The listing builds one solid part. Answer for the finished solid, in the listing's coordinates (mm). Face numbers are marked on the shaded views. A direction names the side the tool comes from. Coordinates: 2 decimals unless noted, no trailing zeros. Order: outer loops, then holes, each group sorted by start corner. A loop starts at its lowest first (then second) coordinate and runs counter-clockwise, first axis right, second up. Notation, with made-up numbers: (24.25, 67) -> (50.25, 67) arc R31 ccw to (50.25, 91) -> close; hole circle Ø1 at (60.25, 74). An arc over 180 degrees is marked (long way). Write each question's results on one line, items separated by ' | '. Start each with the question number.
(1) Given pin 1 (3 mm diameter, centred on y = -1, z = 15, fed in from +X); pin 2 (0.5 mm diameter, centred on x = -17, y = 13.5, fed in from +Z); pin 3 (1 mm diameter, centred on y = 14.5, z = 5.5, fed in from +X); pin 4 (2 mm diameter, centred on x = 19.5, y = -17.5, fed in from -Z), each flat-ended and moving along its own axis, determine where each tip first touches the part or whether it passes through.
(2) The part is cut by section B-B, the plane z = 1. Give the vertices of the cut face in (x, y).
(3) A tool of negligible diameter and unlimited length cuts with its end or side. For the marked faces 1 and 2, from which of +Z, -Z, +X, -X, +Y, -Y can it reach the whole face along a straight path? Write none if from no direction.
(4) The part is cut by section A-A, the plane z = 10.25. Count the separate pieces of the cut face and the enclosed holes in it, then the cut area to 3 significant figures.
(5) Straight lines are drawn through the part: L1, parallel to Y at x = 12, z = 13; L2, parallel to X at y = 19.5, z = 7.75; L3, parallel to Y at x = -3.5, z = 14.25. For each, find the intervals that lie inside material, in ascending order.
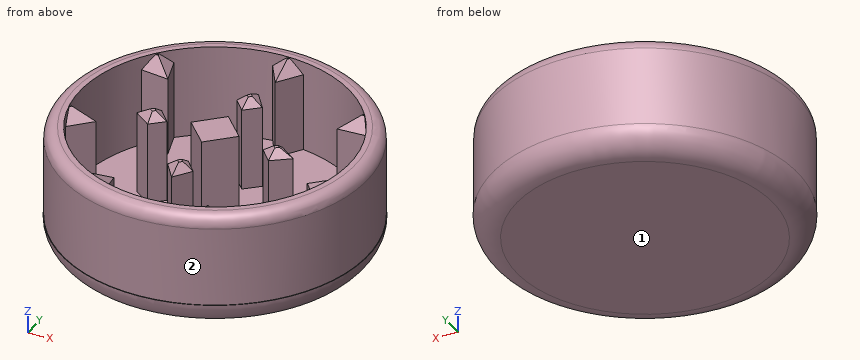
```python
from build123d import *

# Parameters (mm, degrees)
F0_R      = 25
F1_DEPTH  = 4
F3_DEPTH  = 14.8
F4_R      = 24.9
F4_R_2    = 22
F5_DEPTH  = 15
F6_SIZE   = 1.3
F7_SIZE   = 2
F8_R      = 3.99999
F9_R      = 2
F10_R     = 4.5599564507
F11_DEPTH = 0.2


# Not quite as in the source:
# - a fillet or chamfer is up to 0.001 mm smaller than in the source, because OpenCascade refuses the exact size
# - a feature names something its author has since deleted; it is built from what else it names


with BuildPart() as f1:
    # F0 (on Top) → F1 (new body)
    with BuildSketch(Plane.XY):
        Circle(F0_R)
    extrude(amount=F1_DEPTH)

    # F2 (on face) → F3 (join)
    with BuildSketch(Plane.XY.offset(4)):
        Polygon((1.9764285987, -10.1112626395), (0, -8), (-2.2552952007, -10.1112626395), (0, -13), align=None)
        Polygon((0, -4), (4, 0), (0, 4), (-4, 0), align=None)
        Polygon((-10.1112626395, -1.9764285987), (-8, 0), (-10.1112626395, 2.2552952007), (-13, 0), align=None)
        Polygon((-1.9764285987, 10.1112626395), (0, 8), (2.2552952007, 10.1112626395), (0, 13), align=None)
        Polygon((10.1112626395, 1.9764285987), (8, 0), (10.1112626395, -2.2552952007), (13, 0), align=None)
        with BuildLine():
            Line((14.0729666844, 11.2228164335), (18.6727000521, 11.6331540333))
            ThreePointArc((18.6727000521, 11.6331540333), (17.2002926143, 13.7167756409), (15.4965532289, 15.6159161763))
            Line((15.4965532289, 15.6159161763), (14.0729666844, 11.2228164335))
        make_face()
        with BuildLine():
            ThreePointArc((20.7374041193, -7.3457518602), (21.448414068, -4.895460547), (21.8709577964, -2.3793287015))
            Line((21.8709577964, -2.3793287015), (17.5487024193, -4.0053768112))
            Line((17.5487024193, -4.0053768112), (20.7374041193, -7.3457518602))
        make_face()
        with BuildLine():
            ThreePointArc((7.1864199187, -20.793156777), (9.5454422606, -19.8213150939), (11.776085057, -18.5828905376))
            Line((11.776085057, -18.5828905376), (7.8099073041, -16.2174396222))
            Line((7.8099073041, -16.2174396222), (7.1864199187, -20.793156777))
        make_face()
        with BuildLine():
            Line((-7.1864199187, -20.793156777), (-7.8099073041, -16.2174396222))
            Line((-7.8099073041, -16.2174396222), (-11.776085057, -18.5828905376))
            ThreePointArc((-11.776085057, -18.5828905376), (-9.5454422606, -19.8213150939), (-7.1864199187, -20.793156777))
        make_face()
        with BuildLine():
            Line((-20.7374041193, -7.3457518602), (-17.5487024193, -4.0053768112))
            Line((-17.5487024193, -4.0053768112), (-21.8709577964, -2.3793287015))
            ThreePointArc((-21.8709577964, -2.3793287015), (-21.448414068, -4.895460547), (-20.7374041193, -7.3457518602))
        make_face()
        with BuildLine():
            Line((-18.6727000521, 11.6331540333), (-14.0729666844, 11.2228164335))
            Line((-14.0729666844, 11.2228164335), (-15.4965532289, 15.6159161763))
            ThreePointArc((-15.4965532289, 15.6159161763), (-17.2002926143, 13.7167756409), (-18.6727000521, 11.6331540333))
        make_face()
        with BuildLine():
            Line((0, 18), (2.547071992, 21.8520576667))
            ThreePointArc((2.547071992, 21.8520576667), (0, 22), (-2.547071992, 21.8520576667))
            Line((-2.547071992, 21.8520576667), (0, 18))
        make_face()
    extrude(amount=F3_DEPTH)

    # F4 (on face) → F5 (join)
    with BuildSketch(Plane.XY.offset(4)):
        Circle(F4_R)
        Circle(F4_R_2, mode=Mode.SUBTRACT)
    extrude(amount=F5_DEPTH)

    # F6
    f6_edges = [f1.edges().sort_by_distance(p)[0] for p in [
        (-9.055631, -0.988214, 18.8),
        (-9.055631, 1.127648, 18.8),
        (-11.555631, 1.127648, 18.8),
        (-11.555631, -0.988214, 18.8),
        (0.988214, -9.055631, 18.8),
        (-1.127648, -9.055631, 18.8),
        (-1.127648, -11.555631, 18.8),
        (0.988214, -11.555631, 18.8),
        (9.055631, 0.988214, 18.8),
        (9.055631, -1.127648, 18.8),
        (11.555631, -1.127648, 18.8),
        (11.555631, 0.988214, 18.8),
        (-0.988214, 9.055631, 18.8),
        (1.127648, 9.055631, 18.8),
        (1.127648, 11.555631, 18.8),
        (-0.988214, 11.555631, 18.8),
    ]]
    chamfer(f6_edges, length=F6_SIZE)

    # F7
    f7_edges = [f1.edges().sort_by_distance(p)[0] for p in [
        (14.78476, 13.419366, 18.8),
        (16.372833, 11.427985, 18.8),
        (19.70983, -3.192353, 18.8),
        (19.143053, -5.675564, 18.8),
        (9.792996, -17.400165, 18.8),
        (7.498164, -18.505298, 18.8),
        (-9.792996, -17.400165, 18.8),
        (-7.498164, -18.505298, 18.8),
        (-19.143053, -5.675564, 18.8),
        (-19.70983, -3.192353, 18.8),
        (-16.372833, 11.427985, 18.8),
        (-1.273536, 19.926029, 18.8),
        (1.273536, 19.926029, 18.8),
        (-14.78476, 13.419366, 18.8),
    ]]
    chamfer(f7_edges, length=F7_SIZE)

    # F8 (radius 4 in the source; OpenCascade refuses exactly that, so slightly less here)
    f8_edges = [f1.edges().sort_by_distance(p)[0] for p in [
        (-25, 0, 0),
    ]]
    fillet(f8_edges, radius=F8_R)

    # F9
    f9_edges = [f1.edges().sort_by_distance(p)[0] for p in [
        (-24.9, 0, 19),
    ]]
    fillet(f9_edges, radius=F9_R)

    # F10 (on face) → F11 (cut)
    with BuildSketch(Plane.XY.offset(18.8)):
        Circle(F10_R)
    extrude(amount=-F11_DEPTH, mode=Mode.SUBTRACT)


solid = f1.part
```
Established:
1) pin 1: stops at x = 24.9 | pin 2: stops at z = 18.8 | pin 3: stops at x = 20.59 | pin 4: passes through
2) outline: circle Ø47.29 at (0, 0)
3) face 1: -Z, +X, -X, +Y, -Y | face 2: +Z
4) separate pieces: 6 | enclosed holes: 1 | area: 574 mm^2
5) L1: y = -21.82 to -18.44, -0.78 to 0.68, 18.44 to 21.82 | L2: x = -15.48 to -10.19, -0.99 to 0.99, 10.19 to 15.48 | L3: y = -24.65 to -21.72, -0.5 to 0.5, 21.72 to 24.65
